The listing builds one solid part. Answer for the finished solid, in the listing's coordinates (mm). A direction names the side the tool comes from. Coordinates: 2 decimals unless noted, no trailing zeros. Write each loop counter-clockwise with the first axis right and the second up, starting at its lowest first coordinate (ties: lowest second). Pieces come first, ordered by that corner, then holes.
from build123d import *

# Parameters (mm, degrees)
EXTRUDE_1_DEPTH     = 3
SKETCH_2_R          = 2
SKETCH_2_R_2        = 3
CUT_EXTRUDE_1_DEPTH = 10
FILLET_1_R          = 10
FILLET_2_R          = 2
FILLET_3_R          = 3


with BuildPart() as part:
    # 草图1 → 凸台-拉伸1 (new body)
    with BuildSketch(Plane(origin=(0, 0, 0), x_dir=(1, 0, 0), z_dir=(0, 1, 0))):
        with BuildLine():
            Line((-55, 0), (-40, 0))
            Line((-40, 0), (-40, 50.5))
            Line((-40, 50.5), (-132.5, 50.5))
            Line((-132.5, 50.5), (-132.5, 81))
            Line((-132.5, 81), (-211, 81))
            ThreePointArc((-211, 81), (-216.656854249, 78.656854249), (-219, 73))
            Line((-219, 73), (-219, 26))
            Line((-219, 26), (-204, 26))
            Line((-204, 26), (-204, 66))
            Line((-204, 66), (-147.5, 66))
            Line((-147.5, 66), (-147.5, 35.5))
            Line((-147.5, 35.5), (-55, 35.5))
            Line((-55, 35.5), (-55, 0))
        make_face()
    extrude(amount=EXTRUDE_1_DEPTH)

    # 草图2 → 切除-拉伸1 (cut)
    with BuildSketch(Plane(origin=(0, 3, 0), x_dir=(1, 0, 0), z_dir=(0, 1, 0))):
        with Locations(Location((-47.5, 32.5, 0), (0, 0, 270))):
            Circle(SKETCH_2_R)
        with Locations(Location((-211.5, 33.5, 0), (0, 0, 270))):
            Circle(SKETCH_2_R)
        with Locations(Location((-211.5, 48.5, 0), (0, 0, 270))):
            Circle(SKETCH_2_R)
        with Locations(Location((-211, 73, 0), (0, 0, 270))):
            Circle(SKETCH_2_R_2)
        with Locations(Location((-171.5, 73.5, 0), (0, 0, 270))):
            Circle(SKETCH_2_R)
        with Locations(Location((-127, 44.5, 0), (0, 0, 270))):
            Circle(SKETCH_2_R)
        with Locations(Location((-62.5, 43, 0), (0, 0, 270))):
            Circle(SKETCH_2_R)
        with Locations(Location((-47.5, 7.5, 0), (0, 0, 270))):
            Circle(SKETCH_2_R)
    extrude(amount=-CUT_EXTRUDE_1_DEPTH, mode=Mode.SUBTRACT)

    # 圆角1
    fillet_1_edges = [part.edges().sort_by_distance(p)[0] for p in [
        (-147.5, 1.5, -35.5),
        (-132.5, 1.5, -81),
    ]]
    fillet(fillet_1_edges, radius=FILLET_1_R)

    # 圆角2
    fillet_2_edges = [part.edges().sort_by_distance(p)[0] for p in [
        (-40, 1.5, -50.5),
        (-55, 1.5, -35.5),
        (-147.5, 1.5, -66),
        (-132.5, 1.5, -50.5),
    ]]
    fillet(fillet_2_edges, radius=FILLET_2_R)

    # 圆角3
    fillet_3_edges = [part.edges().sort_by_distance(p)[0] for p in [
        (-204, 1.5, -66),
    ]]
    fillet(fillet_3_edges, radius=FILLET_3_R)


solid = part.part
Q1. The part is cut by section D-D, the plane z = -12.5. Write down the section's boundary in (x, y).
Answers below:
outline: (-55, 0) - (-40, 0) - (-40, 3) - (-55, 3) - close
Q2. Given pin 1 (3.5 mm diameter, centred on x = -62.5, z = -43, fed in from +Y); pin 2 (1.5 mm diameter, centred on y = 1, z = -52, fed in from +X), each flat-ended and moving along its own axis, determine where each tip first touches the part or whether it passes through.
Answers below:
pin 1: passes through
pin 2: stops at x = -132.06
Q3. Find the intervals of material crossed by probe 1 along X at (y, z) = (0.4, -28); probe 2 along Z at (x, y) = (-171.5, 1.1); probe 3 along X at (y, z) = (0.95, -43), in increasing order.
Answers below:
probe 1: x = -219 to -204, -55 to -40
probe 2: z = -81 to -75.5, -71.5 to -66
probe 3: x = -219 to -204, -147.18 to -128.32, -125.68 to -64.5, -60.5 to -40
Q4. The part is cut by section C-C, the plane x = -171.5. Write down the section's boundary in (y, z), then the cut area to 3 significant figures.
Answers below:
outline: (0, -81) - (3, -81) - (3, -75.5) - (0, -75.5) - close; (0, -71.5) - (3, -71.5) - (3, -66) - (0, -66) - close
area: 33.0 mm2
Q5. Which of the six approach directions +Z, -Z, +X, -X, +Y, -Y give full straight-line access (tool end or side, diameter ignored) to faces 1 (the face through (-130, 3, -47)), 2 (the face through (-132.5, 1, -62)), 3 (the face through (-98, 1, -35.5))?
Answers below:
face 1: +Z, -Z, +X, -X, +Y
face 2: -Z, +X, +Y, -Y
face 3: +Z, +Y, -Y
Q6. The part is cut by section B-B, the plane z = -55.5. Write down the section's boundary in (x, y).
Answers below:
outline: (-219, 0) - (-204, 0) - (-204, 3) - (-219, 3) - close; (-147.5, 0) - (-132.5, 0) - (-132.5, 3) - (-147.5, 3) - close
Q7. Determine the mould class of faces 4 (the face through (-203.1, 1.52, -65.14)), 5 (the face through (-49.274, 1.521, -31.577)), 6 (the face through (-40, 1, -24)) for opening direction Z: released by +Z, released by -Z, zero draft, split by the parting line, or undercut.
Answers below:
face 4: released by +Z
face 5: undercut
face 6: zero draft
Q8. The part is cut by section A-A, the plane y = 0.5. State how many separate pieces and enclosed holes the cut face has, then the cut area to 3 significant figures.
Answers below:
separate pieces: 1
enclosed holes: 8
area: 4,110 mm2
